from build123d import *

# Parameters (mm, degrees)
SKETCH1_W            = 132
SKETCH1_H            = 95
BOSS_EXTRUDE1_DEPTH  = 5
M5_CLEARANCE_SLOT1_D = 5.3
SKETCH4_W            = 132
SKETCH4_H            = 10
BOSS_EXTRUDE2_DEPTH  = 10
SKETCH5_W            = 100
SKETCH5_H            = 10
SKETCH5_H_2          = 2.5
SKETCH5_W_2          = 16
CUT_EXTRUDE1_DEPTH   = 5


with BuildPart() as part:
    # Sketch1 → Boss-Extrude1 (new body)
    with BuildSketch(Plane(origin=(0, 0, 0), x_dir=(1, 0, 0), z_dir=(0, 1, 0))):
        Rectangle(SKETCH1_W, SKETCH1_H)
    extrude(amount=BOSS_EXTRUDE1_DEPTH)

    # M5 Clearance Slot1 (through all)
    with Locations(Plane(origin=(0, 5, 0), x_dir=(1, 0, 0), z_dir=(0, 1, 0))):
        with Locations((-51, 32.5), (51, 32.5), (51, -32.5), (-51, -32.5)):
            Hole(M5_CLEARANCE_SLOT1_D / 2)

    # Sketch4 → Boss-Extrude2 (add)
    with BuildSketch(Plane(origin=(0, 5, 0), x_dir=(1, 0, 0), z_dir=(0, 1, 0))):
        with Locations((0, 22.5)):
            Rectangle(SKETCH4_W, SKETCH4_H)
        with Locations((0, 42.5)):
            Rectangle(SKETCH4_W, SKETCH4_H)
        with Locations((0, -22.5)):
            Rectangle(SKETCH4_W, SKETCH4_H)
        with Locations((0, -42.5)):
            Rectangle(SKETCH4_W, SKETCH4_H)
    extrude(amount=BOSS_EXTRUDE2_DEPTH)

    # Sketch5 → Cut-Extrude1 (cut)
    with BuildSketch(Plane(origin=(0, 15, 0), x_dir=(1, 0, 0), z_dir=(0, 1, 0))):
        Polygon((-50, -27.5), (-50, -37.5), (50, -37.5), (50, -27.5), (50, -17.5), (50, 17.5), (50, 27.5), (50, 50), (-50, 50), (-50, 27.5), (-50, 17.5), (-50, -17.5), align=None)
        with Locations((0, -42.5)):
            Rectangle(SKETCH5_W, SKETCH5_H)
        with Locations((0, -48.75)):
            Rectangle(SKETCH5_W, SKETCH5_H_2)
        with Locations((-58, -22.5)):
            Rectangle(SKETCH5_W_2, SKETCH5_H)
        with Locations((58, -22.5)):
            Rectangle(SKETCH5_W_2, SKETCH5_H)
        with Locations((58, 22.5)):
            Rectangle(SKETCH5_W_2, SKETCH5_H)
        with Locations((-58, 22.5)):
            Rectangle(SKETCH5_W_2, SKETCH5_H)
    extrude(amount=-CUT_EXTRUDE1_DEPTH, mode=Mode.SUBTRACT)


solid = part.part
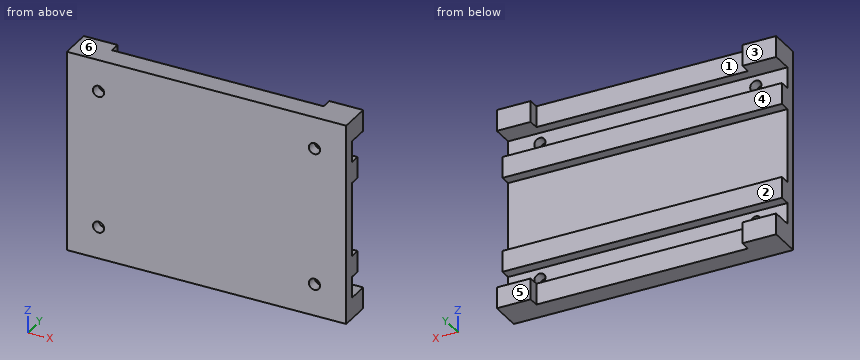
Check sheet for the modelled part. Datum: model origin and axes. Units: mm. Face numbers are marked on the shaded views. A direction names the side the tool comes from. Round coordinates to 2 decimals unless told otherwise and drop trailing zeros. Order: outer loops, then holes, each group sorted by start corner. A loop starts at its lowest first (then second) coordinate and runs counter-clockwise, first axis right, second up. Notation, with made-up numbers: M 1.25,43 L 16.25,43 A23 cw 16.25,67 Z; hole C -14.75,-19 d5. An arc over 180 degrees is marked long. One line per item, written item: value. Start each with the question number.
1. Section check C-C on x = -38. Enter the section's corners in (y, z).
2. Section check D-D on z = 41. Enter the section's corners in (x, y).
3. Release check for a two-part mould opening along Z. For the marked faces 4, 5 and 6 record: released by +Z, released by -Z, zero draft, split by the parting line, or undercut.
4. Access from +Z, -Z, +X, -X, +Y, -Y to the whole of each face (thin tool, end or side, straight path). Record for the marked faces 1, 2 and 3.
5. Section check B-B on z = -32.5. Enter the section's corners in (x, y), and give its area (3 significant figures).
6. Gauge pin test, flat ends, axial feed: P1, Ø8, axis at x = -22.5, z = -7, coming from the +Y side; P2, Ø10, axis at x = 2, z = -34.5, coming from the +Y side; P3, Ø2, axis at x = -16, y = 12.5, coming from the -Z side. Record the tip position at first contact, or that the pin passes through.
7. Scan lines: line 1 along X through (y, z) = (3.2, -32.5); line 2 along Z through (x, y) = (57, 9.75); line 3 along Z through (x, y) = (51, 3.6). Record each from-to range of solid material in increasing order.
8. Section check A-A on y = 8.25. Enter the section's corners in (x, z), and give its area (3 significant figures).
Results found:
1. outline: M 0,-47.5 L 10,-47.5 L 10,-37.5 L 5,-37.5 L 5,-27.5 L 10,-27.5 L 10,-17.5 L 5,-17.5 L 5,17.5 L 10,17.5 L 10,27.5 L 5,27.5 L 5,37.5 L 10,37.5 L 10,47.5 L 0,47.5 Z
2. outline: M -66,0 L 66,0 L 66,15 L 50,15 L 50,10 L -50,10 L -50,15 L -66,15 Z
3. face 4: undercut
3. face 5: zero draft
3. face 6: released by +Z
4. face 1: +Z, -Z, +Y
4. face 2: +X, -X, +Y
4. face 3: +Z, -Z, +X, -X, +Y
5. outline: M -66,0 L -53.65,0 L -53.65,5 L -66,5 Z; M -48.35,0 L 48.35,0 L 48.35,5 L -48.35,5 Z; M 53.65,0 L 66,0 L 66,5 L 53.65,5 Z
5. area: 607 mm^2
6. P1: y = 5
6. P2: y = 10
6. P3: through
7. line 1: -66 to -53.65, -48.35 to 48.35, 53.65 to 66
7. line 2: -47.5 to -37.5, -27.5 to -17.5, 17.5 to 27.5, 37.5 to 47.5
7. line 3: -47.5 to -35.15, -29.85 to 29.85, 35.15 to 47.5
8. outline: M -66,-47.5 L 66,-47.5 L 66,-37.5 L -66,-37.5 Z; M -66,-27.5 L 66,-27.5 L 66,-17.5 L -66,-17.5 Z; M -66,17.5 L 66,17.5 L 66,27.5 L -66,27.5 Z; M -66,37.5 L 66,37.5 L 66,47.5 L -66,47.5 Z
8. area: 5,280 mm^2
